from build123d import *

# Parameters (mm, degrees)
SKETCH2_R           = 67.5
BOSS_EXTRUDE1_DEPTH = 8
SKETCH6_R           = 67.5
SKETCH6_R_2         = 55
BOSS_EXTRUDE2_DEPTH = 10
SKETCH7_R           = 3.3
CUT_EXTRUDE3_DEPTH  = 15
CIRPATTERN2_COUNT   = 6


with BuildPart() as part:
    # Sketch1 → Revolve1 (revolve)
    with BuildSketch(Plane.XY, mode=Mode.PRIVATE) as revolve1_sk:
        with BuildLine():
            Line((-65, 0), (-65, 5))
            Line((-65, 5), (-54.772255751, 5))
            ThreePointArc((-54.772255751, 5), (-37.080992435, 40.620192023), (0, 55))
            Line((0, 55), (0, 50))
            ThreePointArc((0, 50), (-35.355339059, 35.355339059), (-50, 0))
            Line((-50, 0), (-65, 0))
        make_face()
    revolve(revolve1_sk.sketch.rotate(Axis((0, 0, 0), (0, 1, 0)), 180), axis=Axis((0, 0, 0), (0, 1, 0)))

    # Sketch2 → Boss-Extrude1 (add)
    with BuildSketch(Plane(origin=(0, 0, 0), x_dir=(1, 0, 0), z_dir=(0, 1, 0))):
        with Locations(Location((0, 0, 0), (0, 0, 270))):
            Circle(SKETCH2_R)
    extrude(amount=BOSS_EXTRUDE1_DEPTH)

    # Sketch6 → Boss-Extrude2 (add)
    with BuildSketch(Plane(origin=(0, 8, 0), x_dir=(1, 0, 0), z_dir=(0, 1, 0))):
        with Locations(Location((0, 0, 0), (0, 0, 270))):
            Circle(SKETCH6_R)
        with Locations(Location((0, 0, 0), (0, 0, 270))):
            Circle(SKETCH6_R_2, mode=Mode.SUBTRACT)
    extrude(amount=BOSS_EXTRUDE2_DEPTH)

    # Sketch7 → Cut-Extrude3 (cut)
    with BuildSketch(Plane(origin=(0, 18, 0), x_dir=(1, 0, 0), z_dir=(0, 1, 0))):
        with Locations(Location((0, -60, 0), (0, 0, 270))):
            Circle(SKETCH7_R)
    cut_extrude3 = extrude(amount=-CUT_EXTRUDE3_DEPTH, mode=Mode.SUBTRACT)

    # CirPattern2: Cut-Extrude3 ×6 about axis
    cirpattern2_axis = Axis((0, 0, 0), (0, 1, 0))
    for i in range(1, CIRPATTERN2_COUNT):
        add(cut_extrude3.rotate(cirpattern2_axis, i * 360 / CIRPATTERN2_COUNT), mode=Mode.SUBTRACT)


solid = part.part
Verification items for the finished model (mm, model axes). A direction names the side the tool comes from. Give positions to 0.01 mm unless a question says otherwise; leave off trailing zeros. Write each loop counter-clockwise with the first axis right and the second up, starting at its lowest first coordinate (ties: lowest second). Pieces come first, ordered by that corner, then holes.
(1) Cross-section at A-A (x = 0). Enter the section's corners in (y, z).
(2) Access from +Z, -Z, +X, -X, +Y, -Y to the whole of each face (thin tool, end or side, straight path). Record for faces 4 (the face through (-59.884, 8.874, 31.147)), 5 (the face through (-48.74, 10.6, 30.72)).
(3) Cross-section at D-D (x = 47). Enter the section's corners in (y, z).
(4) Cross-section at B-B (z = 0). Enter the section's corners in (x, y).
(5) Gauge pin test, flat ends, axial feed: pin 1 (6 mm diameter, centred on x = 51.96, z = 30, fed in from +Y); pin 2 (8 mm diameter, centred on x = 42, y = 34.5, fed in from -Z); pin 3 (10.5 mm diameter, centred on x = 0, z = -60, fed in from +Y); pin 4 (5 mm diameter, centred on y = 33.5, z = 47, fed in from +X). Record the tip position at first contact, or that the pin passes through.
(6) Material ranges on line 1 (X direction, y = 8.75, z = -30); line 2 (Z direction, x = -3.5, y = 14); line 3 (Y direction, x = 25, z = -59), recorded low to high.
(7) Cross-section at C-C (z = 60). Enter the section's corners in (x, y).
(8) Mould release check, pull along Y, two halves, no side actions. Record for faces 1 (the face through (48.74, 10.6, -30.72)), 2 (the face through (52, 3, 30)), 3 (the face through (1, 8, -1)): +Y half, -Y half, draft (parallel to the pull), parting line (faces both ways), or undercut.
Worked out:
1. outline: (0, -67.5) - (18, -67.5) - (18, -63.3) - (3, -63.3) - (3, -56.7) - (18, -56.7) - (18, -55) - (8, -55) - (8, -54.42) arc R55 ccw to (8, 54.42) - (8, 55) - (18, 55) - (18, 56.7) - (3, 56.7) - (3, 63.3) - (18, 63.3) - (18, 67.5) - (0, 67.5) - close; hole (8, -49.36) arc R50 ccw to (8, 49.36) - close
2. face 4: +Y, -Y
2. face 5: +Y
3. outline: (0, -48.45) - (18, -48.45) - (18, -28.57) - (8, -28.57) - (8, -27.42) arc R28.57 ccw to (8, 27.42) - (8, 28.57) - (18, 28.57) - (18, 48.45) - (0, 48.45) - close; hole (8, -15.07) arc R17.06 ccw to (8, 15.07) - close
4. outline: (-67.5, 0) - (67.5, 0) - (67.5, 18) - (55, 18) - (55, 8) - (54.42, 8) arc R55 ccw to (-54.42, 8) - (-55, 8) - (-55, 18) - (-67.5, 18) - close; hole (-49.36, 8) - (49.36, 8) arc R50 ccw to start
5. pin 1: stops at y = 3
5. pin 2: stops at z = -22.13
5. pin 3: stops at y = 18
5. pin 4: passes through
6. line 1: x = -60.47 to -55.26, -48.66 to -46.1, -45.26 to -39.03, 39.03 to 45.26, 46.1 to 48.66, 55.26 to 60.47
6. line 2: z = -67.41 to -54.89, -53.07 to -47.87, 47.87 to 53.07, 54.89 to 67.41
6. line 3: y = 0 to 18
7. outline: (-30.92, 0) - (30.92, 0) - (30.92, 18) - (3.3, 18) - (3.3, 3) - (-3.3, 3) - (-3.3, 18) - (-30.92, 18) - close
8. face 1: draft
8. face 2: +Y half
8. face 3: undercut
